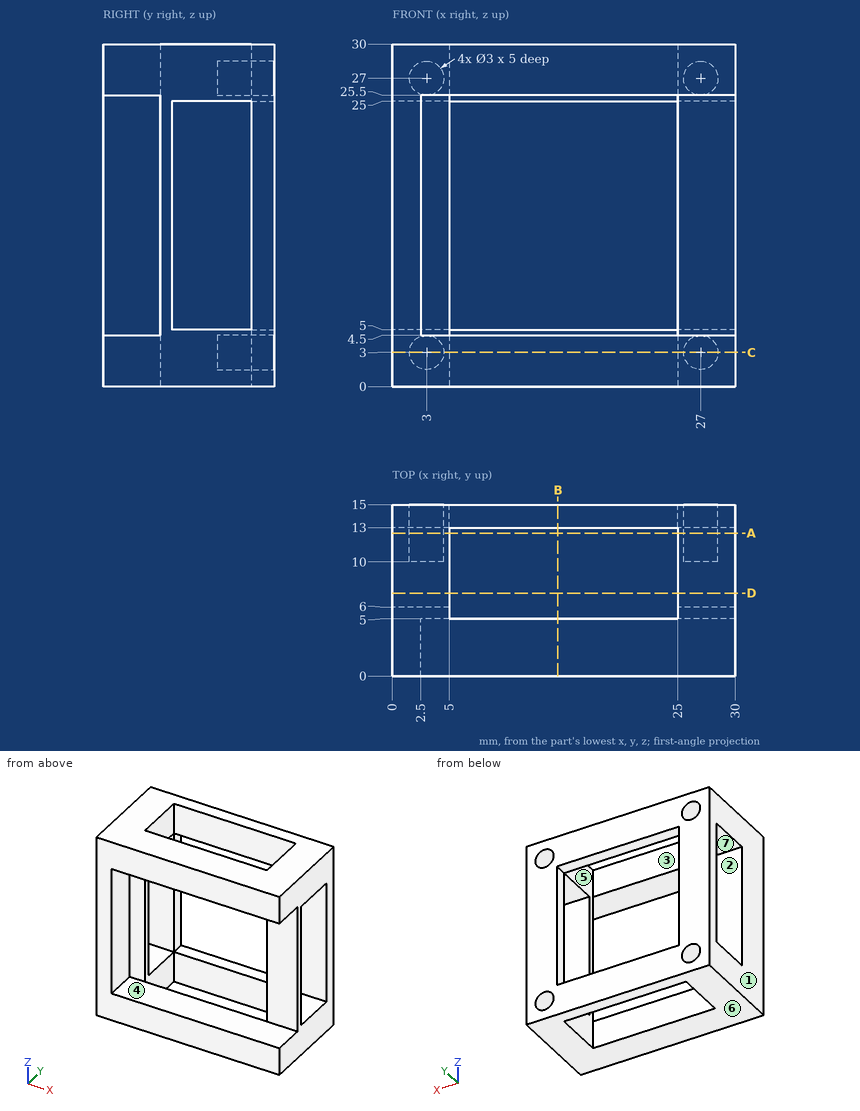
Input: dimensioned drawing with shaded views. Units: mm. Origin: part minimum x, y, z. A direction names the side the tool comes from. Coordinates: 2 decimals unless noted, no trailing zeros. Loops run counter-clockwise (first coordinate to the right, second up) from the corner with the lowest first, then second, coordinate; pieces in that order, holes last. Notation, with made-up numbers: M 27.5,-39 L 65.5,-39 A16 cw 65.5,-15 Z; hole C 45,14 d3. An arc over 180 degrees is marked long. Put each result on its own line as item: value.
(1) First-contact query: pin 1 (2.5 mm diameter, centred on y = 1.5, z = 17, fed in from +X). Flat tip, straight axial feed; report the tip coordinate or a pass-through.
Answer sheet:
pin 1: stops at x = 2.5
(2) Cut plane D-D on y = 7.25. Return the cut outline in (x, z).
Answer sheet:
outline: M 0,0 L 5,0 L 5,5 L 0,5 Z; M 0,25 L 5,25 L 5,30 L 0,30 Z; M 25,0 L 30,0 L 30,5 L 25,5 Z; M 25,25 L 30,25 L 30,30 L 25,30 Z
(3) Cut plane B-B on x = 14.5. Return the cut outline in (y, z), then the cut area to 3 significant figures.
Answer sheet:
outline: M 0,0 L 5,0 L 5,4.5 L 0,4.5 Z; M 0,25.5 L 5,25.5 L 5,30 L 0,30 Z; M 13,0 L 15,0 L 15,5 L 13,5 Z; M 13,25 L 15,25 L 15,30 L 13,30 Z
area: 65.0 mm^2
(4) Material intervals for probe 1 along X at (y, z) = (12.4, 3); probe 2 along X at (y, z) = (13.9, 3); probe 3 along X at (y, z) = (14.25, 9.75), sorted ascending.
Answer sheet:
probe 1: x = 0 to 1.5, 4.5 to 5, 25 to 25.5, 28.5 to 30
probe 2: x = 0 to 1.5, 4.5 to 25.5, 28.5 to 30
probe 3: x = 0 to 5, 25 to 30
(5) Draft query along Z for the marked faces 5, 6 and 7. Return one class per face: pulls with the +Z half, pulls with the -Z half, needs draft (parallel to the pull), parting line crosses it, or undercut.
Answer sheet:
face 5: needs draft
face 6: pulls with the -Z half
face 7: undercut
(6) Access query for the marked faces 1, 2, 3 and 4. Directions: +Z, -Z, +X, -X, +Y, -Y. A direction counts if a zero-diameter tool reaches every point of the face in a straight line with its end or side. Return the directions, or none.
Answer sheet:
face 1: +Z, -Z, -X, +Y, -Y
face 2: +X, -X
face 3: +Z, -Z
face 4: +X, -Y
(7) Cut plane C-C on z = 3. Return the cut outline in (x, y), then the cut area to 3 significant figures.
Answer sheet:
outline: M 0,0 L 30,0 L 30,15 L 28.5,15 L 28.5,10 L 25.5,10 L 25.5,15 L 4.5,15 L 4.5,10 L 1.5,10 L 1.5,15 L 0,15 Z; hole M 5,5 L 25,5 L 25,13 L 5,13 Z
area: 260 mm^2
(8) Cut plane A-A on y = 12.5. Return the cut outline in (x, z), then the cut area to 3 significant figures.
Answer sheet:
outline: M 0,0 L 5,0 L 5,5 L 0,5 Z; M 0,25 L 5,25 L 5,30 L 0,30 Z; M 25,0 L 30,0 L 30,5 L 25,5 Z; M 25,25 L 30,25 L 30,30 L 25,30 Z; hole C 3,3 d3; hole C 3,27 d3; hole C 27,3 d3; hole C 27,27 d3
area: 71.7 mm^2
